Check sheet for the drawn part. Datum: minimum x, y, z corner. Units: mm. A direction names the side the tool comes from. Round coordinates to 2 decimals unless told otherwise and drop trailing zeros. Order: outer loops, then holes, each group sorted by start corner. A loop starts at its lowest first (then second) coordinate and runs counter-clockwise, first axis right, second up.
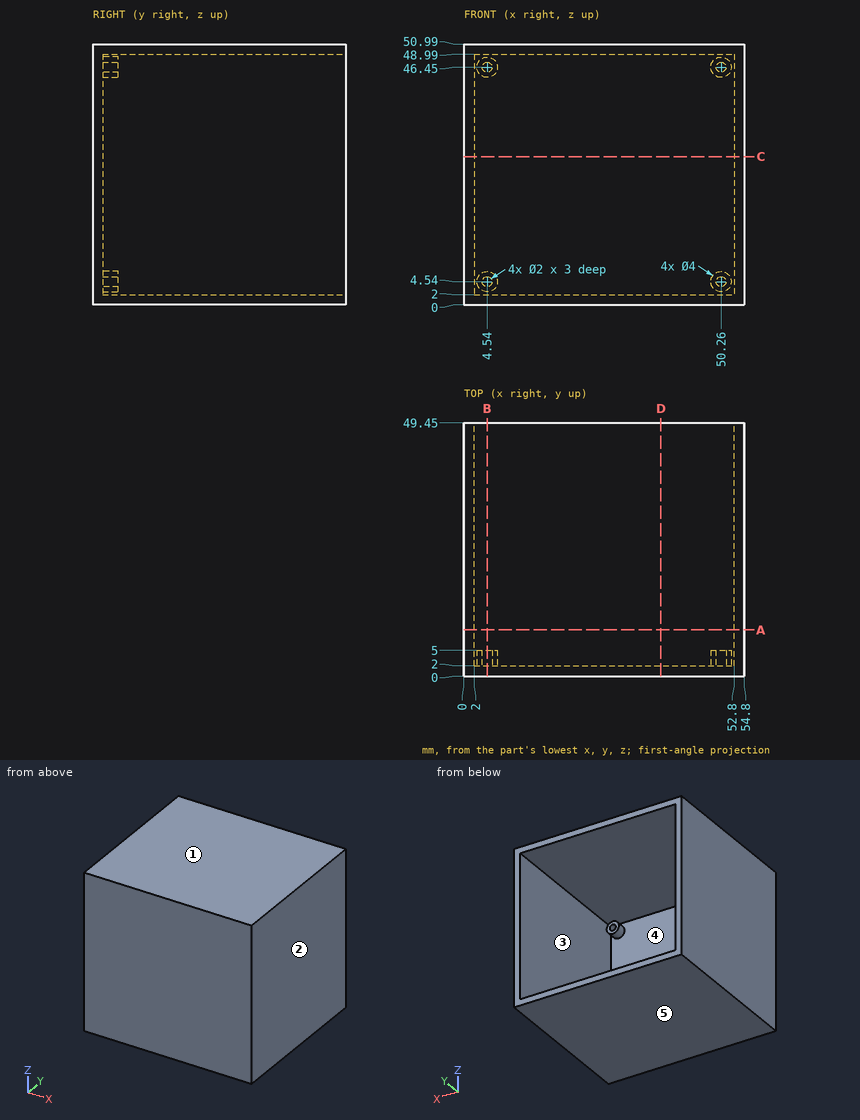
(1) Draft check along X on the marked faces 1, 2 and 3. Enter one of: released by +X, released by -X, zero draft, split by the parting line, or undercut.
Returned:
face 1: zero draft
face 2: released by +X
face 3: undercut
(2) Sectioned sample at D-D, the plane x = 38.5. Record the cut outline in (y, z), and give its area (3 significant figures).
Returned:
outline: (0, 0) - (49.45, 0) - (49.45, 2) - (2, 2) - (2, 48.99) - (49.45, 48.99) - (49.45, 50.99) - (0, 50.99) - close
area: 292 mm2
(3) Depth check by flat-ended pin: P1, Ø1.2, axis at x = 51, z = 45.5, coming from the +Y side; P2, Ø12, axis at x = 20, z = 22, coming from the +Y side. Enter the tip coordinate at first touch or a pass-through.
Returned:
P1: stops at y = 5
P2: stops at y = 2
(4) Sectioned sample at B-B, the plane x = 4.54. Record the cut outline in (y, z).
Returned:
outline: (0, 0) - (49.45, 0) - (49.45, 2) - (2, 2) - (2, 2.54) - (5, 2.54) - (5, 3.54) - (2, 3.54) - (2, 5.54) - (5, 5.54) - (5, 6.54) - (2, 6.54) - (2, 44.45) - (5, 44.45) - (5, 45.45) - (2, 45.45) - (2, 47.45) - (5, 47.45) - (5, 48.45) - (2, 48.45) - (2, 48.99) - (49.45, 48.99) - (49.45, 50.99) - (0, 50.99) - close
(5) Sectioned sample at A-A, the plane y = 9. Record the cut outline in (x, z), and give its area (3 significant figures).
Returned:
outline: (0, 0) - (54.8, 0) - (54.8, 50.99) - (0, 50.99) - close; hole (2, 2) - (52.8, 2) - (52.8, 48.99) - (2, 48.99) - close
area: 407 mm2
(6) Material ranges on line 1 (X direction, y = 3.9, z = 46.45); line 2 (Z direction, x = 21, y = 18); line 3 (X direction, y = 29, z = 42.5), recorded low to high.
Returned:
line 1: x = 0 to 2, 2.54 to 3.54, 5.54 to 6.54, 48.26 to 49.26, 51.26 to 52.26, 52.8 to 54.8
line 2: z = 0 to 2, 48.99 to 50.99
line 3: x = 0 to 2, 52.8 to 54.8
(7) Set-up check for the marked faces 4 and 5: record each of +Z, -Z, +X, -X, +Y, -Y from which the full face is reachable in a straight line by a thin tool's end or side.
Returned:
face 4: +Y
face 5: -Z, +X, -X, +Y, -Y
(8) Sectioned sample at C-C, the plane z = 29. Record the cut outline in (x, y), and give its area (3 significant figures).
Returned:
outline: (0, 0) - (54.8, 0) - (54.8, 49.45) - (52.8, 49.45) - (52.8, 2) - (2, 2) - (2, 49.45) - (0, 49.45) - close
area: 299 mm2
